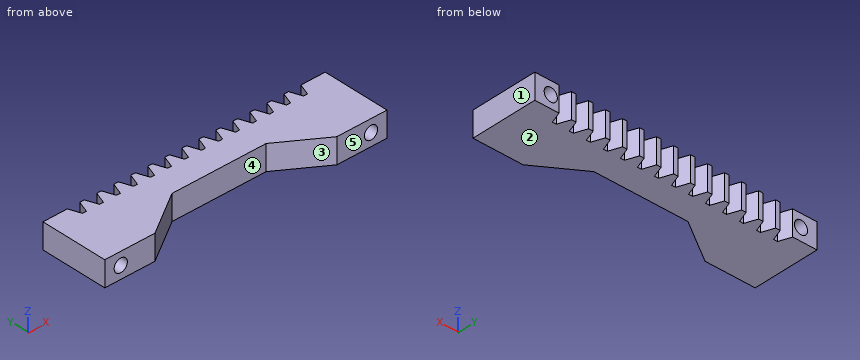
```python
from build123d import *

# Parameters (mm, degrees)
SKETCH3_W           = 45
SKETCH3_H           = 10.6
BOSS_EXTRUDE2_DEPTH = 4
CUT_EXTRUDE4_REACH  = 44.658
SKETCH4_R           = 1.05
CUT_EXTRUDE7_REACH  = 44.513
CUT_EXTRUDE8_START  = -4
CUT_EXTRUDE8_DEPTH  = 4


# Read off the part's stored shape, not the designer's step: Cut-Extrude8
with BuildPart() as part:
    # Sketch3 → Boss-Extrude2 (new body)
    with BuildSketch(Plane.XY):
        with Locations((-18.626321401, 4.7)):
            Rectangle(SKETCH3_W, SKETCH3_H)
    extrude(amount=-BOSS_EXTRUDE2_DEPTH)

    # Sketch4 → Cut-Extrude4 (cut, up to next)
    with BuildSketch(Plane(origin=(0, 10, 0), x_dir=(1, 0, 0), z_dir=(0, 1, 0)), mode=Mode.PRIVATE) as cut_extrude4_sk1:
        with Locations(Location((-38.576321401, 2, 0), (0, 0, 180))):
            Circle(SKETCH4_R)
    cut_extrude4_tool1 = extrude(cut_extrude4_sk1.sketch, amount=-CUT_EXTRUDE4_REACH, mode=Mode.PRIVATE) & part.part
    # Sketch4 → Cut-Extrude4 (cut, up to next)
    with BuildSketch(Plane(origin=(0, 10, 0), x_dir=(1, 0, 0), z_dir=(0, 1, 0)), mode=Mode.PRIVATE) as cut_extrude4_sk2:
        with Locations(Location((1.323678599, 2, 0), (0, 0, 180))):
            Circle(SKETCH4_R)
    cut_extrude4_tool2 = extrude(cut_extrude4_sk2.sketch, amount=-CUT_EXTRUDE4_REACH, mode=Mode.PRIVATE) & part.part
    add(cut_extrude4_tool1.solids().sort_by_distance((-38.576321, 10, -2))[0], mode=Mode.SUBTRACT)
    add(cut_extrude4_tool2.solids().sort_by_distance((1.323679, 10, -2))[0], mode=Mode.SUBTRACT)

    # Sketch6 → Cut-Extrude7 (cut, up to next)
    with BuildSketch(Plane(origin=(0, 0, -4), x_dir=(-1, 0, 0), z_dir=(0, 0, -1)), mode=Mode.PRIVATE) as cut_extrude7_sk1:
        Polygon((4.126321401, -0.6), (11.126321401, 4), (26.126321401, 4), (33.126321401, -0.6), align=None)
    cut_extrude7_tool1 = extrude(cut_extrude7_sk1.sketch, amount=-CUT_EXTRUDE7_REACH, mode=Mode.PRIVATE) & part.part
    add(cut_extrude7_tool1.solids().sort_by_distance((-18.626321, 1.456061, -4))[0], mode=Mode.SUBTRACT)

    # Cut-Extrude8 outline → Cut-Extrude8 (cut)
    with BuildSketch(Plane.XY.offset(CUT_EXTRUDE8_START)):
        Polygon((-35.264703894, 10), (-37.252642802, 10), (-36.571857508, 8.129557778), (-35.945489188, 8.129557778), align=None)
        Polygon((0, 10), (-1.987938907, 10), (-1.307153614, 8.129557778), (-0.680785294, 8.129557778), align=None)
        Polygon((-2.71266953, 10), (-4.700608438, 10), (-4.019823144, 8.129557778), (-3.393454824, 8.129557778), align=None)
        Polygon((-5.425339061, 10), (-7.413277968, 10), (-6.732492674, 8.129557778), (-6.106124354, 8.129557778), align=None)
        Polygon((-8.138008591, 10), (-10.125947498, 10), (-9.445162205, 8.129557778), (-8.818793885, 8.129557778), align=None)
        Polygon((-10.850678121, 10), (-12.838617029, 10), (-12.157831735, 8.129557778), (-11.531463415, 8.129557778), align=None)
        Polygon((-13.563347652, 10), (-15.551286559, 10), (-14.870501265, 8.129557778), (-14.244132945, 8.129557778), align=None)
        Polygon((-16.276017182, 10), (-18.263956089, 10), (-17.583170796, 8.129557778), (-16.956802476, 8.129557778), align=None)
        Polygon((-18.988686712, 10), (-20.97662562, 10), (-20.295840326, 8.129557778), (-19.669472006, 8.129557778), align=None)
        Polygon((-21.701356243, 10), (-23.68929515, 10), (-23.008509856, 8.129557778), (-22.382141536, 8.129557778), align=None)
        Polygon((-24.414025773, 10), (-26.40196468, 10), (-25.721179387, 8.129557778), (-25.094811067, 8.129557778), align=None)
        Polygon((-27.126695303, 10), (-29.114634211, 10), (-28.433848917, 8.129557778), (-27.807480597, 8.129557778), align=None)
        Polygon((-29.839364834, 10), (-31.827303741, 10), (-31.146518447, 8.129557778), (-30.520150127, 8.129557778), align=None)
        Polygon((-32.552034364, 10), (-34.539973271, 10), (-33.859187978, 8.129557778), (-33.232819658, 8.129557778), align=None)
    extrude(amount=CUT_EXTRUDE8_DEPTH, mode=Mode.SUBTRACT)


solid = part.part
```
CAD build for the part. Positions are in the model's coordinates, mm. Face numbers are marked on the shaded views. A direction names the side the tool comes from. Coordinates: 2 decimals unless noted, no trailing zeros. Loops run counter-clockwise (first coordinate to the right, second up) from the corner with the lowest first, then second, coordinate; pieces in that order, holes last. Notation, with made-up numbers: (-2, -27.5) - (9, -27.5) arc R24 cw to (9, 7.5) - close; hole circle Ø6 at (9.25, -24.75). An arc over 180 degrees is marked (long way). Use CSV: the item, a comma, the result in double quotes. Start each with the question number.
Q1. Cut at B-B, the plane y = 7.5. List the corners of the cut face in (x, z), then the cut area to 3 significant figures.
Q2. Cut at A-A, the plane y = 1. List the corners of the cut face in (x, z), then the cut area to 3 significant figures.
Q3. Probe probe 1 along X at (y, z) = (4.5, -1.1); probe 2 along X at (y, z) = (0, -1.8); probe 3 along X at (y, z) = (3.75, -1.55) (3 decimals). List the from-to ranges inside material, lowest first. Write a range as from..to.
Q4. Two-plate mould, pull along X, no slides. Class the marked faces 1, 2 and 3: +X half, -X half, draft (parallel to the pull), parting line (faces both ways), or undercut.
Q5. 3-axis set-ups, long thin cutter, end or side, ignore diameter. For the marked faces 4 and 5: which of +Z, -Z, +X, -X, +Y, -Y reach the whole face in a straight line?
Q6. Cut at C-C, the plane z = -2. State how many separate pieces and enclosed holes the cut face has, then the cut area to 3 significant figures.
Q7. Drop flat-ended pins along their axis: P1, Ø2, axis at x = -20.5, z = -1.5, coming from the -Y side; P2, Ø1.5, axis at x = -30, z = -1.5, coming from the -Y side. Give the stop position or say it passes through.
Here are the results:
1,outline,"(-41.13, -4) - (3.87, -4) - (3.87, 0) - (-41.13, 0) - close; hole circle Ø2.1 at (-38.58, -2); hole circle Ø2.1 at (1.32, -2)"
1,area,"173 mm2"
2,outline,"(-41.13, -4) - (-30.69, -4) - (-30.69, 0) - (-41.13, 0) - close; (-6.56, -4) - (3.87, -4) - (3.87, 0) - (-6.56, 0) - close; hole circle Ø2.1 at (-38.58, -2); hole circle Ø2.1 at (1.32, -2)"
2,area,"76.6 mm2"
3,probe 1,"-41.13..-39.12, -38.04..0.78, 1.86..3.87"
3,probe 2,"-41.13..-39.61, -37.55..-32.21, -5.04..0.29, 2.35..3.87"
3,probe 3,"-41.126..-39.525, -37.628..-26.507, -10.746..0.375, 2.272..3.874"
4,face 1,"+X half"
4,face 2,"draft"
4,face 3,"undercut"
5,face 4,"+Z, -Z, -Y"
5,face 5,"+Z, -Z, +X, -X, -Y"
6,separate pieces,"3"
6,enclosed holes,"0"
6,area,"297 mm2"
7,P1,"y = 4"
7,P2,"y = 0.96"
